Check sheet for the modelled part. Datum: model origin and axes. Units: mm. A direction names the side the tool comes from. Round coordinates to 2 decimals unless told otherwise and drop trailing zeros. Write each loop counter-clockwise with the first axis right and the second up, starting at its lowest first coordinate (ties: lowest second). Pieces come first, ordered by that corner, then holes. Notation, with made-up numbers: (-14.75, 28.5) -> (23.25, 28.5) arc R25 cw to (23.25, 42.5) -> close; hole circle Ø9 at (6, 80). An arc over 180 degrees is marked (long way). Write item = value, one per line.
from build123d import *

# Parameters (mm, degrees)
SKETCH_3_W      = 78
SKETCH_3_H      = 78
SKETCH_3_R      = 4.25
EXTRUDE_1_DEPTH = 5
EXTRUDE_2_DEPTH = 3.5
SKETCH_5_W      = 78
SKETCH_5_H      = 78
SKETCH_5_R      = 4.25
EXTRUDE_3_DEPTH = 5


with BuildPart() as part:
    # 草图3 → 凸台-拉伸1 (new body)
    with BuildSketch(Plane.XY):
        with Locations((0, 39)):
            Rectangle(SKETCH_3_W, SKETCH_3_H)
        with Locations((-20, 61.45)):
            Circle(SKETCH_3_R, mode=Mode.SUBTRACT)
        with Locations(Location((20, 61.45, 0), (0, 0, 180))):
            Circle(SKETCH_3_R, mode=Mode.SUBTRACT)
        with BuildLine():
            Line((-15.75, 39.75), (-15.75, 22.25))
            ThreePointArc((-15.75, 22.25), (-20, 18), (-24.25, 22.25))
            Line((-24.25, 22.25), (-24.25, 39.75))
            ThreePointArc((-24.25, 39.75), (-20, 44), (-15.75, 39.75))
        make_face(mode=Mode.SUBTRACT)
        with BuildLine():
            Line((15.75, 39.75), (15.75, 22.25))
            ThreePointArc((15.75, 22.25), (20, 18), (24.25, 22.25))
            Line((24.25, 22.25), (24.25, 39.75))
            ThreePointArc((24.25, 39.75), (20, 44), (15.75, 39.75))
        make_face(mode=Mode.SUBTRACT)
    extrude(amount=EXTRUDE_1_DEPTH)

    # 草图4 → 凸台-拉伸2 (add)
    with BuildSketch(Plane.ZY.offset(39)):
        Polygon((5, 78), (8.5, 78), (8.5, 69.8), (69.8, 8.5), (78, 8.5), (78, 0), (5, 0), align=None)
    extrude_2 = extrude(amount=-EXTRUDE_2_DEPTH)

    # 镜向1: 凸台-拉伸2 across plane
    add(extrude_2.mirror(Plane(origin=(0, 0, 0), x_dir=(0, 0, 1), z_dir=(1, 0, 0))))

    # 草图5 → 凸台-拉伸3 (add)
    with BuildSketch(Plane.XZ):
        with Locations((0, 39)):
            Rectangle(SKETCH_5_W, SKETCH_5_H)
        with Locations((-20, 61.414216079)):
            Circle(SKETCH_5_R, mode=Mode.SUBTRACT)
        with Locations(Location((20, 61.414216079, 0), (0, 0, 180))):
            Circle(SKETCH_5_R, mode=Mode.SUBTRACT)
        with BuildLine():
            Line((-15.75, 39.714216079), (-15.75, 22.214216079))
            ThreePointArc((-15.75, 22.214216079), (-20, 17.964216079), (-24.25, 22.214216079))
            Line((-24.25, 22.214216079), (-24.25, 39.714216079))
            ThreePointArc((-24.25, 39.714216079), (-20, 43.964216079), (-15.75, 39.714216079))
        make_face(mode=Mode.SUBTRACT)
        with BuildLine():
            Line((15.75, 39.714216079), (15.75, 22.214216079))
            ThreePointArc((15.75, 22.214216079), (20, 17.964216079), (24.25, 22.214216079))
            Line((24.25, 22.214216079), (24.25, 39.714216079))
            ThreePointArc((24.25, 39.714216079), (20, 43.964216079), (15.75, 39.714216079))
        make_face(mode=Mode.SUBTRACT)
    extrude(amount=-EXTRUDE_3_DEPTH)


solid = part.part
(1) Sectioned sample at D-D on z = 48. Enter the section's corners in (x, y).
Worked answers:
outline = (-39, 0) -> (39, 0) -> (39, 30.3) -> (35.5, 30.3) -> (35.5, 5) -> (-35.5, 5) -> (-35.5, 30.3) -> (-39, 30.3) -> close
(2) Go/stop test with flat-tipped pins: P1, Ø1, axis at x = 37, z = 76, coming from the +Y side; P2, Ø5, axis at x = -20, z = 61.41, coming from the -Y side; P3, Ø8, axis at x = -5, z = 38, coming from the +Y side; P4, Ø1.5, axis at x = 4.5, y = 48, coming from the +Z side. Record where each tip stops, or that it passes through.
Worked answers:
P1 = 8.5
P2 = through
P3 = 5
P4 = 5
(3) Sectioned sample at C-C on z = 63.5. Enter the section's corners in (x, y).
Worked answers:
outline = (-39, 0) -> (-23.7, 0) -> (-23.7, 5) -> (-35.5, 5) -> (-35.5, 14.8) -> (-39, 14.8) -> close; (-16.3, 0) -> (16.3, 0) -> (16.3, 5) -> (-16.3, 5) -> close; (23.7, 0) -> (39, 0) -> (39, 14.8) -> (35.5, 14.8) -> (35.5, 5) -> (23.7, 5) -> close
(4) Sectioned sample at B-B on y = 46.5. Enter the section's corners in (x, z), then the cut area to 3 significant figures.
Worked answers:
outline = (-39, 0) -> (39, 0) -> (39, 31.8) -> (35.5, 31.8) -> (35.5, 5) -> (-35.5, 5) -> (-35.5, 31.8) -> (-39, 31.8) -> close
area = 578 mm²
(5) Access from +Z, -Z, +X, -X, +Y, -Y to the whole of each face (thin tool, end or side, straight path). Record for faces 1 (the flat face through (24.25, 31, 2)), 2 (the flat face through (35.5, 26, 26)), 3 (the flat face through (37, 74, 8.5)), 4 (the flat face through (24.25, 2, 31)).
Worked answers:
face_1 = +Z, -Z
face_2 = +Z, +Y
face_3 = +Z, +X, -X, +Y
face_4 = +Y, -Y
(6) Material ranges on L1, parallel to Y at x = 20, z = 3.05; L2, parallel to X at y = 20, z = 31.5; L3, parallel to Z at x = -20, y = 2, recorded low to high. Write a range as [from, to].
Worked answers:
L1 = [0, 18], [44, 57.2], [65.7, 78]
L2 = [-39, -35.5], [35.5, 39]
L3 = [0, 17.96], [43.96, 57.16], [65.66, 78]
(7) Release check for a two-part mould opening along X. For faces 5 (the flat face through (-15.75, 31, 2)), 6 (the flat face through (39, 22, 22)), 7 (the flat face through (37.3, 39.6, 38.7)) record: pulls with the +X half, pulls with the -X half, needs draft (parallel to the pull), parting line crosses it, or undercut.
Worked answers:
face_5 = undercut
face_6 = pulls with the +X half
face_7 = needs draft
(8) Sectioned sample at A-A on x = -20. Enter the section's corners in (y, z).
Worked answers:
outline = (0, 0) -> (18, 0) -> (18, 5) -> (5, 5) -> (5, 17.96) -> (0, 17.96) -> close; (0, 43.96) -> (5, 43.96) -> (5, 57.16) -> (0, 57.16) -> close; (0, 65.66) -> (5, 65.66) -> (5, 78) -> (0, 78) -> close; (44, 0) -> (57.2, 0) -> (57.2, 5) -> (44, 5) -> close; (65.7, 0) -> (78, 0) -> (78, 5) -> (65.7, 5) -> close
